The model under review builds one solid part; all positions refer to its coordinate system, in mm. Coordinates: 2 decimals unless noted, no trailing zeros. Loops run counter-clockwise (first coordinate to the right, second up) from the corner with the lowest first, then second, coordinate; pieces in that order, holes last. Notation, with made-up numbers: M 23,-38.5 L 81,-38.5 A21 cw 81,-15.5 Z; hole C -37.75,18 d9. An arc over 180 degrees is marked long. Use one line per item in the form item = value.
Autodesk Fusion 360 part; units mm, degrees
sketch "Sketch1" plane through (0, 0, 0) normal (0, 1, 0) x (1, 0, 0)
  circle A0 centre (0, 0) radius 17.095
  circle A1 centre (0, 0) radius 32.5
  line L0 (-21.05, 0) -> (0, 0)
  line L1 (0, 0) -> (-19.4454, 19.4454)
  circle A2 centre (-19.4454, 19.4454) radius 0.5
  circle A3 centre (-19.4454, -19.4454) radius 0.5
  circle A4 centre (19.4454, -19.4454) radius 0.5
  circle A5 centre (19.4454, 19.4454) radius 0.5
  line L2 (17.3241, -8.1317) -> (8.1317, -17.3241)
  line L3 (0, 0) -> (12.7279, -12.7279)
  line L4 (10.253, -19.4454) -> (8.1317, -17.3241)
  line L5 (8.1317, -17.3241) -> (11.3137, -14.1421)
  line L6 (11.3137, -14.1421) -> (13.435, -16.2635)
  line L7 (13.435, -16.2635) -> (10.253, -19.4454)
  line L8 (19.4454, -10.253) -> (17.3241, -8.1317)
  line L9 (17.3241, -8.1317) -> (14.1421, -11.3137)
  line L10 (14.1421, -11.3137) -> (16.2635, -13.435)
  line L11 (16.2635, -13.435) -> (19.4454, -10.253)
  line L12 (11.844, -17.8544) -> (13.6118, -19.6222)
  circle A6 centre (13.6118, -19.6222) radius 0.5
  line L13 (17.8544, -11.844) -> (19.6222, -13.6118)
  circle A7 centre (19.6222, -13.6118) radius 0.5
  circle A8 centre (-13.6118, 19.6222) radius 0.5
  circle A9 centre (-19.6222, 13.6118) radius 0.5
  dimension "d1" = 34.19
  dimension "d4" = 21.05
  dimension "d7" = 27.5
  dimension "d8" = 1
  dimension "d9" = 45
  dimension "d13" = 13
  dimension "d14" = 18
  dimension "d15" = 3
  dimension "d16" = 4.5
  dimension "d18" = 4.5
  dimension "d19" = 2.5
  dimension "d20" = 1
  dimension "d21" = 2.5
  dimension "d22" = 1
  dimension "d24" = 360
  dimension "d27" = 65
extrude "Extrude1" add sketch "Sketch1" along normal blind 2 contours L2 L8 L9 L10 L11 | L2 L4 L5 L6 L7 | A1
1. Wall thickness on line 1 along X through (y, z) = (1.15, 0) (3 decimals); line 2 along Z through (x, y) = (0.5, 1.85); line 3 along Z through (x, y) = (19.5, 1.85): over which ranges is each line inside the solid? List them lowest first. Write a range as from..to.
Response values:
line_1 = -32.5..-17.095, 17.095..32.5
line_2 = -32.5..-17.09, 17.09..32.5
line_3 = -26..-19.94, -18.95..13.13, 14.1..18.95, 19.94..26
2. The part is to be moulded in two halves that separate along X. For faces 1 (the face through (31, 0.99, 9.76)), 2 (the face through (-2.23, 0.99, 16.95)), 3 (the face through (14, 2, 14)), say which applies: pulls with the +X half, pulls with the -X half, needs draft (parallel to the pull), parting line crosses it, or undercut.
Response values:
face_1 = parting line crosses it
face_2 = undercut
face_3 = needs draft
3. Insertion check: P1, Ø1, axis at x = -6.5, y = 1, coming from the -Z side; P2, Ø1, axis at y = 1.5, z = 13.5, coming from the +X side; P3, Ø10, axis at x = -18.5, z = -18.5, coming from the -Y side; P4, Ø1, axis at x = -1, y = 0, coming from the -Z side. Each pin has a flat end and moves straight along its axis. Give the tip position at first contact, or say it passes through.
Response values:
P1 = -31.94
P2 = 29.79
P3 = 0
P4 = -32.5
4. Add section C-C (y = 0.35). Count the separate pieces of the cut face and the enclosed holes in it, then the cut area to 3 significant figures.
Response values:
separate_pieces = 1
enclosed_holes = 9
area = 2,390 mm^2
5. Add section D-D (z = -26). State the section outline as (x, y) points, then the cut area to 3 significant figures.
Response values:
outline = M -19.5,0 L 19.5,0 L 19.5,2 L -19.5,2 Z
area = 78.0 mm^2
6. Add section B-B (z = 0). State the section outline as (x, y) points (3 decimals), then the cut area to 3 significant figures.
Response values:
outline = M -32.5,0 L -17.095,0 L -17.095,2 L -32.5,2 Z; M 17.095,0 L 32.5,0 L 32.5,2 L 17.095,2 Z
area = 61.6 mm^2
7. Add section A-A (x = 0). State the section outline as (y, z) points (3 decimals).
Response values:
outline = M 0,-32.5 L 2,-32.5 L 2,-17.095 L 0,-17.095 Z; M 0,17.095 L 2,17.095 L 2,32.5 L 0,32.5 Z
